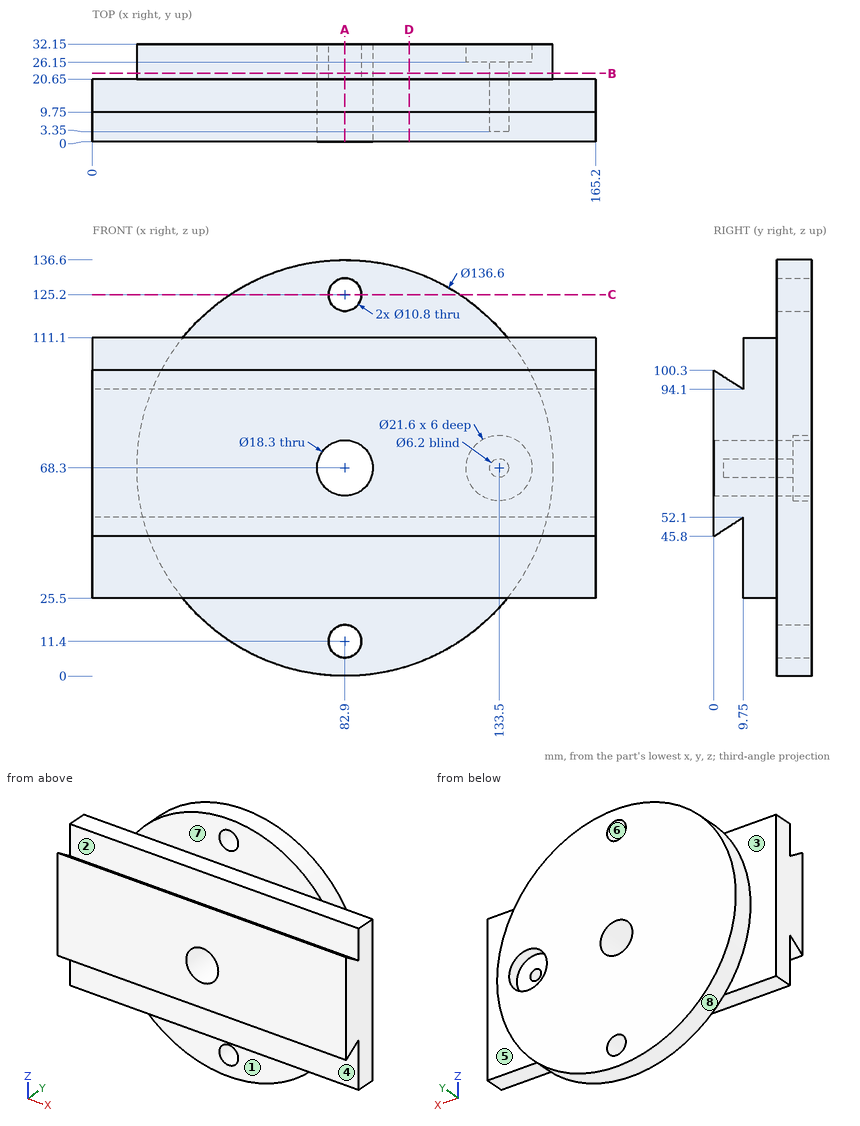
Geometry: see drawing. Coordinates: mm, zero at the bounding-box minimum. A direction names the side the tool comes from. Give positions to 0.01 mm unless a question says otherwise; leave off trailing zeros. Loops run counter-clockwise (first coordinate to the right, second up) from the corner with the lowest first, then second, coordinate; pieces in that order, holes last. Notation, with made-up numbers: (52.5, -18) - (79.5, -18) arc R27 ccw to (79.5, 6) - close; hole circle Ø6 at (53, -38). An arc over 180 degrees is marked (long way). Use CSV: the item, a comma, the result in double quotes.
1) Cut plane A-A (x = 82.9). Output: boundary loops of the cut face in (y, z).
Worked out:
outline,"(0, 45.8) - (9.75, 52.1) - (9.75, 25.5) - (20.65, 25.5) - (20.65, 16.8) - (32.15, 16.8) - (32.15, 59.15) - (0, 59.15) - close; (0, 77.45) - (32.15, 77.45) - (32.15, 119.8) - (20.65, 119.8) - (20.65, 111.1) - (9.75, 111.1) - (9.75, 94.1) - (0, 100.3) - close; (20.65, 0) - (32.15, 0) - (32.15, 6) - (20.65, 6) - close; (20.65, 130.6) - (32.15, 130.6) - (32.15, 136.6) - (20.65, 136.6) - close"
2) Cut plane C-C (z = 125.2). Output: boundary loops of the cut face in (x, y), and give its area (3 significant figures).
Worked out:
outline,"(45.12, 20.65) - (77.5, 20.65) - (77.5, 32.15) - (45.12, 32.15) - close; (88.3, 20.65) - (120.68, 20.65) - (120.68, 32.15) - (88.3, 32.15) - close"
area,"745 mm^2"
3) Set-up query: the marked faces 1, 2, 3, 4 and 5. Return all of +Z, -Z, +X, -X, +Y, -Y with unobstructed straight access to the full face (end or side cutting, diameter ignored); none if empty.
Worked out:
face 1,"-Z, +X, -X, -Y"
face 2,"+Z, +X, -X"
face 3,"-X, +Y"
face 4,"-Z, +X, -X"
face 5,"+X, +Y"
4) Mould query, pull axis Z, two halves, no side actions, for the marked faces 6, 7 and 8. Classes: +Z half, -Z half, draft (parallel to the pull), parting line (faces both ways), or undercut.
Worked out:
face 6,"undercut"
face 7,"draft"
face 8,"parting line"
5) Pin query (flat end, axial travel): P1, Ø1, axis at x = 64, y = 28, coming from the +Z side; P2, Ø4, axis at x = 109, y = 17, coming from the -Z side; P3, Ø10, axis at x = 26.5, y = 11, coming from the +Z side; P4, Ø14.5, axis at x = 82.9, z = 68.3, coming from the +Y side. Return the tip coordinate at first contact, or that it passes through.
Worked out:
P1,"stops at z = 134.07"
P2,"stops at z = 25.5"
P3,"stops at z = 111.1"
P4,"passes through"
6) Line query: line 1 (X direction, y = 17.5, z = 68.3); line 2 (X direction, y = 27, z = 68); line 3 (Z direction, x = 82.9, y = 29). Output: solid intervals per line, ascending.
Worked out:
line 1,"x = 0 to 73.75, 92.05 to 130.4, 136.6 to 165.2"
line 2,"x = 14.6 to 73.75, 92.05 to 122.7, 144.3 to 151.2"
line 3,"z = 0 to 6, 16.8 to 59.15, 77.45 to 119.8, 130.6 to 136.6"
7) Cut plane D-D (x = 104). Output: boundary loops of the cut face in (y, z), and give its area (3 significant figures).
Worked out:
outline,"(0, 45.8) - (9.75, 52.1) - (9.75, 25.5) - (20.65, 25.5) - (20.65, 3.34) - (32.15, 3.34) - (32.15, 133.26) - (20.65, 133.26) - (20.65, 111.1) - (9.75, 111.1) - (9.75, 94.1) - (0, 100.3) - close"
area,"2,900 mm^2"
8) Cut plane B-B (y = 22.5). Output: boundary loops of the cut face in (x, z).
Worked out:
outline,"circle Ø136.6 at (82.9, 68.3); hole circle Ø18.3 at (82.9, 68.3); hole circle Ø10.8 at (82.9, 11.4); hole circle Ø10.8 at (82.9, 125.2); hole circle Ø6.2 at (133.5, 68.3)"
